from build123d import *

# Parameters (mm, degrees)
F0_R        = 1.25
F0_R_2      = 30
F0_R_3      = 27.5
F1_DEPTH    = 0.5
F2_R        = 2
F3_R        = 5
F4_R        = 200
F5_T1_DEPTH = 35.8886959127
F6_T1_DEPTH = 56.2497974387
F6_T3_DEPTH = 89.6754808083
F6_T5_DEPTH = 45.7004795966
F6_T7_DEPTH = 39.8671139621
F6_T9_DEPTH = 53.963301214


# Not quite as in the source:
# - a fillet or chamfer that OpenCascade refuses, or shapes differently, is made with other operations: its cross-section is extruded or revolved along the edge and cut away or added


with BuildPart() as f1:
    # F0 (on Front) → F1 (new body)
    with BuildSketch(Plane.XZ):
        Polygon((24, 85), (24, 0), (330, 0), (326, 40), (316, 70), (300, 90), (277, 110), (261, 120), (236, 129), (235, 103), (215, 110), (185, 120), (146, 130), (70, 140), (0, 142), (0, 85), align=None)
        with Locations((35, 10)):
            Circle(F0_R, mode=Mode.SUBTRACT)
        with Locations((75.7, 10)):
            Circle(F0_R, mode=Mode.SUBTRACT)
        with Locations((116.4, 10)):
            Circle(F0_R, mode=Mode.SUBTRACT)
        with Locations((157.1, 10)):
            Circle(F0_R, mode=Mode.SUBTRACT)
        with Locations((97, 65)):
            Circle(F0_R_2, mode=Mode.SUBTRACT)
        with Locations((197.8, 10)):
            Circle(F0_R, mode=Mode.SUBTRACT)
        with Locations((238.5, 10)):
            Circle(F0_R, mode=Mode.SUBTRACT)
        with Locations((279.2, 10)):
            Circle(F0_R, mode=Mode.SUBTRACT)
        with Locations((319.9, 10)):
            Circle(F0_R, mode=Mode.SUBTRACT)
        with Locations((166, 65)):
            Circle(F0_R_3, mode=Mode.SUBTRACT)
    extrude(amount=F1_DEPTH)

    # F2
    f2_edges = [f1.edges().sort_by_distance(p)[0] for p in [
        (24, -0.25, 85),
    ]]
    fillet(f2_edges, radius=F2_R)

    # F3
    f3_edges = [f1.edges().sort_by_distance(p)[0] for p in [
        (235, -0.25, 103),
        (236, -0.25, 129),
    ]]
    fillet(f3_edges, radius=F3_R)

    # F4
    f4_edges = [f1.edges().sort_by_distance(p)[0] for p in [
        (70, -0.25, 140),
        (146, -0.25, 130),
    ]]
    fillet(f4_edges, radius=F4_R)

    # F5: fillet of radius 200 on 1 edges, made by hand

    # F5_s2 → F5_t1 (cut)
    with BuildSketch(Plane.XZ.offset(-17.6943479563)):
        with BuildLine():
            ThreePointArc((178.1440498006, 121.7579359486), (184.9646346256, 119.8799020084), (191.7145329504, 117.7618223499))
            Line((191.7145329504, 117.7618223499), (185, 120))
            Line((185, 120), (178.1440498006, 121.7579359486))
        make_face()
    extrude(amount=F5_T1_DEPTH, mode=Mode.SUBTRACT)

    # F6: fillet of radius 100 on 5 edges, made by hand

    # F6_s2 → F6_t1 (cut)
    with BuildSketch(Plane.XZ.offset(-27.8748987193)):
        with BuildLine():
            ThreePointArc((322.47407322, 50.57778034), (325.3940178786, 39.8703898792), (327.109462436, 28.9053756404))
            Line((327.109462436, 28.9053756404), (326, 40))
            Line((326, 40), (322.47407322, 50.57778034))
        make_face()
    extrude(amount=F6_T1_DEPTH, mode=Mode.SUBTRACT)

    # F6_s4 → F6_t3 (cut)
    with BuildSketch(Plane.XZ.offset(-44.5877404042)):
        with BuildLine():
            ThreePointArc((304.8585037552, 83.9268703061), (314.6138472293, 69.2458956516), (321.6399526159, 53.0801421523))
            Line((321.6399526159, 53.0801421523), (316, 70))
            Line((316, 70), (304.8585037552, 83.9268703061))
        make_face()
    extrude(amount=F6_T3_DEPTH, mode=Mode.SUBTRACT)

    # F6_s6 → F6_t5 (cut)
    with BuildSketch(Plane.XZ.offset(-22.6002397983)):
        with BuildLine():
            ThreePointArc((293.1782936984, 95.9319185231), (299.7058017999, 89.7176239908), (305.6473031502, 82.9408710622))
            Line((305.6473031502, 82.9408710622), (300, 90))
            Line((300, 90), (293.1782936984, 95.9319185231))
        make_face()
    extrude(amount=F6_T5_DEPTH, mode=Mode.SUBTRACT)

    # F6_s8 → F6_t7 (cut)
    with BuildSketch(Plane.XZ.offset(-19.683556981)):
        with BuildLine():
            ThreePointArc((270.3233508253, 114.1729057342), (276.8158857708, 109.7512495983), (282.9413283175, 104.83362755))
            Line((282.9413283175, 104.83362755), (277, 110))
            Line((277, 110), (270.3233508253, 114.1729057342))
        make_face()
    extrude(amount=F6_T7_DEPTH, mode=Mode.SUBTRACT)

    # F6_s10 → F6_t9 (cut)
    with BuildSketch(Plane.XZ.offset(-26.731650607)):
        with BuildLine():
            ThreePointArc((250.9394105782, 123.6218121919), (260.7509863663, 119.487225172), (270.0673577512, 114.3329014055))
            Line((270.0673577512, 114.3329014055), (261, 120))
            Line((261, 120), (250.9394105782, 123.6218121919))
        make_face()
    extrude(amount=F6_T9_DEPTH, mode=Mode.SUBTRACT)


solid = f1.part
Design review of the part built by this model. Coordinates are the model's own, in mm. A direction names the side the tool comes from. Round coordinates to 2 decimals unless told otherwise and drop trailing zeros. Write each loop counter-clockwise with the first axis right and the second up, starting at its lowest first coordinate (ties: lowest second). Pieces come first, ordered by that corner, then holes. Notation, with made-up numbers: (-0.75, 3.25) -> (39.25, 3.25) arc R16 cw to (39.25, 24.25) -> close; hole circle Ø1 at (10.5, 34.5). An arc over 180 degrees is marked (long way). One line per question, with ' | ' between items.
(1) Take a section at C-C, the plane z = 24.5. State the section outline as (x, y) points, and give its area (3 significant figures).
Result sheet:
outline: (24, -0.5) -> (327.55, -0.5) -> (327.55, 0) -> (24, 0) -> close | area: 152 mm2
(2) Take a section at D-D, the plane x = 254.5. State the section outline as (y, z) points, and give its area (3 significant figures).
Result sheet:
outline: (-0.5, 0) -> (0, 0) -> (0, 122.26) -> (-0.5, 122.26) -> close | area: 61.1 mm2
(3) Take a section at B-B, the plane y = -0.25. State how many separate pieces and enclosed holes the cut face has, and give its area (3 significant figures).
Result sheet:
separate pieces: 1 | enclosed holes: 10 | area: 32,500 mm2
(4) Insertion check: P1, Ø2, axis at x = 319.9, z = 10, coming from the +Y side. The pin has a flat end and moves straight along its axis. Give the tip position at first contact, or say it passes through.
Result sheet:
P1: through
(5) Wall thickness on line 1 (Z direction, x = 157.1, y = -0.25); line 2 (X direction, y = -0.3, z = 56.5); line 3 (Z direction, x = 116.4, y = -0.15): over which ranges is each line inside the solid? List them lowest first. Write a range as [from, to].
Result sheet:
line 1: [0, 8.75], [11.25, 38.98], [91.02, 127.15] | line 2: [24, 68.23], [125.77, 139.85], [192.15, 320.43] | line 3: [0, 8.75], [11.25, 42.12], [87.88, 133.89]
(6) Draft analysis for pull direction Z (two halves, no side actions). For faces 3 (the cylindrical face through (314.65, -0.25, 69.18)), 4 (the cylindrical face through (192.23, -0.25, 73.26)), 5 (the flat face through (199, -0.5, 72)), state which applies: released by +Z, released by -Z, zero draft, split by the parting line, or undercut.
Result sheet:
face 3: released by +Z | face 4: undercut | face 5: zero draft
(7) Take a section at A-A, the plane x = 166.5. State the section outline as (y, z) points.
Result sheet:
outline: (-0.5, 0) -> (0, 0) -> (0, 37.5) -> (-0.5, 37.5) -> close; (-0.5, 92.5) -> (0, 92.5) -> (0, 124.74) -> (-0.5, 124.74) -> close
(8) Machinability: for faces 1 (the flat face through (203.52, -0.246, 113.827)), 2 (the cylindrical face through (260.62, -0.25, 119.55)), which of the approach directions +Z, -Z, +X, -X, +Y, -Y give a long, thin tool a straight path to every point of the face, cutting with its end or side? Answer none if there is none.
Result sheet:
face 1: +Z, +Y, -Y | face 2: +Z, +X, +Y, -Y
